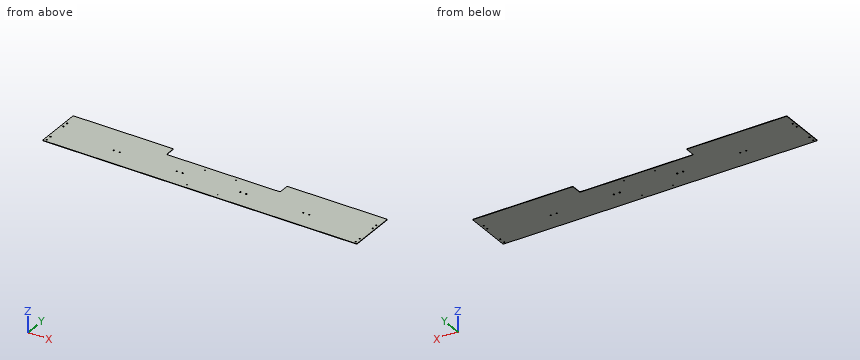
```python
from build123d import *

# Parameters (mm, degrees)
BOSS_EXTRUDE1_DEPTH              = 1.5875
F_25_64_0_39063_DIAMETER_HOLE1_D = 9.922002
FILLET1_R                        = 6.35
F_1_4_CLEARANCE_HOLE2_D          = 6.7564


with BuildPart() as part:
    # Sketch1 → Boss-Extrude1 (new, symmetric)
    with BuildSketch(Plane.XY):
        Polygon((-431.8, 222.25), (-1193.8, 222.25), (-1193.8, 139.7), (-1193.8, -139.7), (1193.8, -139.7), (1193.8, 139.7), (1193.8, 222.25), (431.8, 222.25), (431.8, 139.7), (-431.8, 139.7), align=None)
    extrude(amount=BOSS_EXTRUDE1_DEPTH, both=True)

    # 25/64 (0.39063) Diameter Hole1 (through all)
    with Locations(Plane.XY.offset(1.5875)):
        with Locations((-1174.75, 120.65), (-1174.75, -120.65), (1174.75, 120.65), (1174.75, -120.65), (-742.95, 0), (-698.5, 0), (-263.525, 0), (-219.075, 0), (742.95, 0), (698.5, 0), (263.525, 0), (219.075, 0), (1174.75, -76.2), (1174.75, 76.2), (-1174.75, 76.2), (-1174.75, -76.2)):
            Hole(F_25_64_0_39063_DIAMETER_HOLE1_D / 2)

    # Fillet1
    fillet1_edges = [part.edges().sort_by_distance(p)[0] for p in [
        (1193.8, -139.7, 0),
        (-1193.8, -139.7, 0),
        (-1193.8, 222.25, 0),
        (-431.8, 222.25, 0),
        (-431.8, 139.7, 0),
        (431.8, 139.7, 0),
        (431.8, 222.25, 0),
        (1193.8, 222.25, 0),
    ]]
    fillet(fillet1_edges, radius=FILLET1_R)

    # 1/4 Clearance Hole2 (through all)
    with Locations(Plane.XY.offset(1.5875)):
        with Locations((-117.475, 107.95), (-117.475, -107.95), (117.475, 107.95), (117.475, -107.95)):
            Hole(F_1_4_CLEARANCE_HOLE2_D / 2)


solid = part.part
```
Geometry: final body of the model. Coordinates: model frame, mm. Round coordinates to 2 decimals unless told otherwise and drop trailing zeros. Order: outer loops, then holes, each group sorted by start corner. A loop starts at its lowest first (then second) coordinate and runs counter-clockwise, first axis right, second up. Notation, with made-up numbers: (36, 10) - (85, 10) arc R14 cw to (85, 14) - close; hole circle Ø4 at (-2.75, -29.75). An arc over 180 degrees is marked (long way). Write item = value, one per line. Start each with the question number.
Q1. Cut plane B-B on x = 395. Return the cut outline in (y, z), and give its area (3 significant figures).
Q2. Cut plane A-A on z = -0.4. Give the number of separate pieces and of enclosed holes in the cut face, and give its area (3 significant figures).
Q3. Ray query, line 1 (X direction, y = 107.5, z = 0.7); line 2 (X direction, y = 193, z = -0.75); line 3 (X direction, y = 117, z = -0.7). Return the intervals inside material, ascending. Write a range as from..to.
Q4. Pin query (flat end, axial travel): pin 1 (8 mm diameter, centred on x = 742.95, y = 0, fed in from -Z). Return the tip coordinate at first contact, or that it passes through.
Outcome:
q1.outline = (-139.7, -1.59) - (139.7, -1.59) - (139.7, 1.59) - (-139.7, 1.59) - close
q1.area = 887 mm^2
q2.separate_pieces = 1
q2.enclosed_holes = 20
q2.area = 791,000 mm^2
q3.line_1 = -1193.8..-120.82, -114.13..114.13, 120.82..1193.8
q3.line_2 = -1193.8..-431.8, 431.8..1193.8
q3.line_3 = -1193.8..-1178.11, -1171.39..1171.39, 1178.11..1193.8
q4.pin_1 = through
